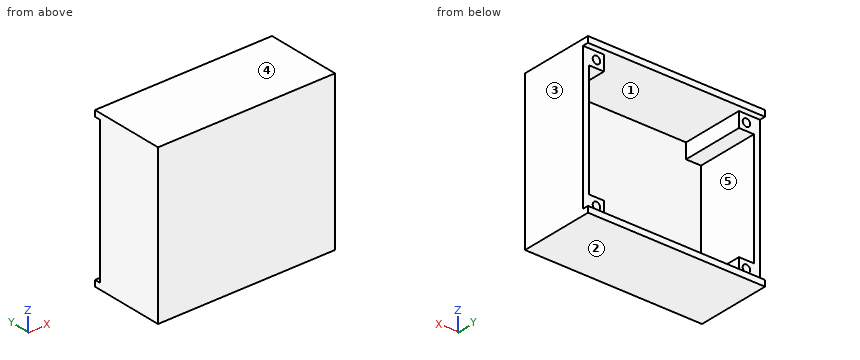
```python
from build123d import *

# Parameters (mm, degrees)
SKETCH1_W               = 118
SKETCH1_H               = 104
SKETCH1_W_2             = 110
SKETCH1_H_2             = 96
BOSS_EXTRUDE1_DEPTH     = 50
SKETCH1_2_W             = 118
SKETCH1_2_H             = 104
BOSS_EXTRUDE2_DEPTH     = 4
SKETCH2_W               = 96
SKETCH2_H               = 4
CUT_EXTRUDE1_DEPTH      = 1
CUT_EXTRUDE1_DEPTH_BACK = 119
SKETCH3_W               = 10
SKETCH3_H               = 10
BOSS_EXTRUDE3_DEPTH     = 42
SKETCH4_R               = 2.5
CUT_EXTRUDE2_DEPTH      = 10


with BuildPart() as part:
    # Sketch1 → Boss-Extrude1 (new body)
    with BuildSketch(Plane(origin=(0, 0, 0), x_dir=(1, 0, 0), z_dir=(0, 1, 0))):
        Rectangle(SKETCH1_W, SKETCH1_H)
        Rectangle(SKETCH1_W_2, SKETCH1_H_2, mode=Mode.SUBTRACT)
    extrude(amount=BOSS_EXTRUDE1_DEPTH)

    # Sketch1<2> → Boss-Extrude2 (add)
    with BuildSketch(Plane(origin=(0, 0, 0), x_dir=(1, 0, 0), z_dir=(0, 1, 0))):
        Rectangle(SKETCH1_2_W, SKETCH1_2_H)
    extrude(amount=BOSS_EXTRUDE2_DEPTH)

    # Sketch2 → Cut-Extrude1 (cut, two sides)
    with BuildSketch(Plane(origin=(59, 0, 0), x_dir=(0, 0, -1), z_dir=(1, 0, 0))) as cut_extrude1_sk:
        with Locations((0, 48)):
            Rectangle(SKETCH2_W, SKETCH2_H)
    extrude(amount=CUT_EXTRUDE1_DEPTH, mode=Mode.SUBTRACT)
    extrude(cut_extrude1_sk.sketch, amount=-CUT_EXTRUDE1_DEPTH_BACK, mode=Mode.SUBTRACT)

    # Sketch3 → Boss-Extrude3 (add)
    with BuildSketch(Plane(origin=(0, 4, 0), x_dir=(1, 0, 0), z_dir=(0, 1, 0))):
        with Locations((-50, 43)):
            Rectangle(SKETCH3_W, SKETCH3_H)
        with Locations((-50, -43)):
            Rectangle(SKETCH3_W, SKETCH3_H)
        with Locations((50, -43)):
            Rectangle(SKETCH3_W, SKETCH3_H)
        with Locations((50, 43)):
            Rectangle(SKETCH3_W, SKETCH3_H)
    extrude(amount=BOSS_EXTRUDE3_DEPTH)

    # Sketch4 → Cut-Extrude2 (cut)
    with BuildSketch(Plane(origin=(0, 46, 0), x_dir=(1, 0, 0), z_dir=(0, 1, 0))):
        with Locations((-50, 43)):
            Circle(SKETCH4_R)
        with Locations((50, 43)):
            Circle(SKETCH4_R)
        with Locations((50, -43)):
            Circle(SKETCH4_R)
        with Locations((-50, -43)):
            Circle(SKETCH4_R)
    extrude(amount=-CUT_EXTRUDE2_DEPTH, mode=Mode.SUBTRACT)


solid = part.part
```
The listing builds one solid part. Answer for the finished solid, in the listing's coordinates (mm). Face numbers are marked on the shaded views. A direction names the side the tool comes from. Coordinates: 2 decimals unless noted, no trailing zeros. Write each loop counter-clockwise with the first axis right and the second up, starting at its lowest first coordinate (ties: lowest second). Pieces come first, ordered by that corner, then holes. Notation, with made-up numbers: (-13.5, 40) - (3.5, 40) arc R24 cw to (3.5, 63) - close; hole circle Ø5 at (84.25, 86.5). An arc over 180 degrees is marked (long way). Return JSON: item names as keys, results as strings. Group by question number.
1. A cutting plane is placed at A-A, the plane y = 22.5. Determine the outline of the cut face in (x, z).
2. Determine the mould class of the marked faces 3, 4 and 5 for opening direction Z: released by +Z, released by -Z, zero draft, split by the parting line, or undercut.
3. Straight lines are drawn through the part: L1, parallel to X at y = 43, z = 43; L2, parallel to Z at x = 50, y = 42.25; L3, parallel to Z at x = 41, y = 11.5. For each, find the intervals that lie inside material, in ascending order.
4. A cutting plane is placed at D-D, the plane x = 25.5. Determine the outline of the cut face in (y, z).
5. A cutting plane is placed at B-B, the plane x = -50. Determine the outline of the cut face in (y, z).
6. Which of the six approach directions +Z, -Z, +X, -X, +Y, -Y give full straight-line access (tool end or side, diameter ignored) to the marked faces 1 and 2?
7. Given pin 1 (10 mm diameter, centred on x = -26, z = 35, fed in from +Y); pin 2 (2.5 mm diameter, centred on x = 50.5, z = -42, fed in from +Y), each flat-ended and moving along its own axis, determine where each tip first touches the part or whether it passes through.
8. A cutting plane is placed at C-C, the plane z = 43. Determine the outline of the cut face in (x, y), plus the area to 3 significant figures.
Ans:
{
 "1": {"outline": "(-59, -52) - (59, -52) - (59, 52) - (-59, 52) - close; hole (-55, -38) - (-45, -38) - (-45, -48) - (45, -48) - (45, -38) - (55, -38) - (55, 38) - (45, 38) - (45, 48) - (-45, 48) - (-45, 38) - (-55, 38) - close"},
 "2": {"face 3": "zero draft", "face 4": "released by +Z", "face 5": "undercut"},
 "3": {"L1": "-59 to -52.5, -47.5 to -45, 45 to 47.5, 52.5 to 59", "L2": "-52 to -45.5, -40.5 to -38, 38 to 40.5, 45.5 to 52", "L3": "-52 to -48, 48 to 52"},
 "4": {"outline": "(0, -52) - (50, -52) - (50, -48) - (4, -48) - (4, 48) - (50, 48) - (50, 52) - (0, 52) - close"},
 "5": {"outline": "(0, -52) - (50, -52) - (50, -48) - (46, -48) - (46, -45.5) - (36, -45.5) - (36, -40.5) - (46, -40.5) - (46, -38) - (4, -38) - (4, 38) - (46, 38) - (46, 40.5) - (36, 40.5) - (36, 45.5) - (46, 45.5) - (46, 48) - (50, 48) - (50, 52) - (0, 52) - close"},
 "6": {"face 1": "+Y", "face 2": "-Z, +X, -X, +Y, -Y"},
 "7": {"pin 1": "y = 4", "pin 2": "y = 36"},
 "8": {"outline": "(-59, 0) - (59, 0) - (59, 46) - (52.5, 46) - (52.5, 36) - (47.5, 36) - (47.5, 46) - (45, 46) - (45, 4) - (-45, 4) - (-45, 46) - (-47.5, 46) - (-47.5, 36) - (-52.5, 36) - (-52.5, 46) - (-59, 46) - close", "area": "1,550 mm²"}
}
